Here's how the part is built. I have some questions about the finished solid (model axes, mm). A direction names the side the tool comes from. Round coordinates to 2 decimals unless told otherwise and drop trailing zeros. Loops run counter-clockwise (first coordinate to the right, second up) from the corner with the lowest first, then second, coordinate; pieces in that order, holes last. Notation, with made-up numbers: M 24.25,-9.5 L 82.25,-9.5 A20 ccw 82.25,26.5 Z; hole C 29,-6 d2. An arc over 180 degrees is marked long. One line per question, with ' | ' between items. Start each with the question number.
Autodesk Inventor part; units mm, degrees
ref_plane "YZ Plane" through (0, 0, 0) normal (1, 0, 0) x (0, 1, 0)
ref_plane "XZ Plane" through (0, 0, 0) normal (0, 1, 0) x (-1, 0, 0)
ref_plane "XY Plane" through (0, 0, 0) normal (0, 0, 1) x (1, 0, 0)
sketch "Sketch2" plane through (0, 0, 0) normal (0, 0, 1) x (1, 0, 0)
  line L0 (-6.9834, -3.25) -> (-3.5959, -3.25)
  arc A0 (-3.5959, -3.25) -> (-3.5959, 3.25) centre (-0.4834, 0) ccw
  circle A1 centre (-6.9834, 0) radius 3.25
  line L1 (7.6359, 0) -> (-9.8597, 0) construction
  line L2 (-6.9834, 3.25) -> (-3.5959, 3.25)
  circle A2 centre (-6.9834, 0) radius 3.25
  circle A3 centre (-0.4834, 0) radius 3.25
  point P0 (-7.0471, -3.1146)
  dimension "d6" = 6.5
  dimension "d7" = 9
  dimension "d8" = 6.5
extrude "Extrusion1" add sketch "Sketch2" along normal blind 10 contours A3 | A1 L2 A0 L0 | A1
extrude "Extrusion2" add sketch "Sketch2" against normal blind 5 contours A3
sketch "Sketch3" plane through (0, 0, 10) normal (0, 0, 1) x (1, 0, 0)
  arc A0 (-6.9834, 3.25) -> (-6.9834, -3.25) centre (-6.9834, 0) ccw
  line L0 (-3.5959, 3.25) -> (-6.9834, 3.25)
  arc A1 (-3.5959, -3.25) -> (-3.5959, 3.25) centre (-0.4834, 0) ccw
  line L1 (-6.9834, -3.25) -> (-3.5959, -3.25)
  circle A2 centre (-6.9834, 0) radius 3.25
  point P0 (-6.9834, -3.25)
  point P1 (-6.9834, 3.25)
  point P2 (-4.0488, -2.7456)
  point P3 (4.0134, -0.1685)
  dimension "d9" = 6.5
extrude "Extrusion3" add sketch "Sketch3" along normal blind 5 contours A2 A0
equation "\"d6\" = R"
equation "\"d7\" = R1"
equation "\"d0\" = 2 * thickness"
equation "\"d2\" = thickness"
equation "\"d9\" = R"
equation "\"R\" = 6.5"
equation "\"thickness\" = 5"
equation "\"width\" = 6.5"
equation "\"R1\" = 9"
1) Imagine slicing it at D-D (x = -4). Write out the boundary of the cut face in (y, z), then the cut area to 3 significant figures.
2) Imagine slicing it at C-C (z = 3.5). Write out the boundary of the cut face in (x, y).
3) Imagine slicing it at A-A (y = 0). Write out the boundary of the cut face in (x, z), then the cut area to 4 significant figures.
4) I'm going to push flat-ended pins straight in: pin 1 Ø3.5 at (x, z) = (-4.5, 7.5) entering from +Y; pin 2 Ø4.5 at (x, y) = (-5.5, 2) entering from -Z; pin 3 Ø1 at (x, y) = (-3.5, 3) entering from +Z; pin 4 Ø2.5 at (x, z) = (-5.5, 4.5) entering from -Y. Where does each tip first touch, or does it pass through?
5) For faces 1 (the face through (-10.23, -0.14, 9.06)), 2 (the face through (-1, 0, -5)), 3 (the face through (-5, 0, 0)), 4 (the face through (-5, -3.25, 5)), 5 (the face through (-5, 3.25, 5)), which set-ups out of +Z, -Z, +X, -X, +Y, -Y let a thin tool reach every point of the face, with its end or its side?
6) Imagine slicing it at B-B (x = 2.25). Write out the boundary of the cut face in (y, z).
7) Please list where these lines run through material, in increasing order: L1, parallel to Z at x = 0.75, y = 2; L2, parallel to Z at x = -7.25, y = -2; L3, parallel to Y at x = -7, z = 11.5. Write a range as from..to.
Results are:
1) outline: M -3.25,0 L 3.25,0 L 3.25,10 L 1.29,10 L 1.29,15 L -1.29,15 L -1.29,10 L -3.25,10 Z | area: 77.9 mm²
2) outline: M -6.98,-3.25 L -3.6,-3.25 A4.5 ccw long -3.6,3.25 L -6.98,3.25 A3.25 ccw Z
3) outline: M -10.23,0 L -3.73,0 L -3.73,-5 L 2.77,-5 L 2.77,0 L 4.02,0 L 4.02,10 L -3.73,10 L -3.73,15 L -10.23,15 Z | area: 207.5 mm²
4) pin 1: y = 3.89 | pin 2: z = -5 | pin 3: z = 10 | pin 4: y = -3.25
5) face 1: +Z | face 2: -Z, +X, -X, +Y, -Y | face 3: -Z | face 4: +Z, -Z, -X, -Y | face 5: +Z, -Z, -X, +Y
6) outline: M -3.57,0 L -1.76,0 L -1.76,-5 L 1.76,-5 L 1.76,0 L 3.57,0 L 3.57,10 L -3.57,10 Z
7) L1: -5..10 | L2: 0..15 | L3: -3.25..3.25
